Autodesk Inventor part; units mm, degrees
ref_plane "YZ Plane" through (0, 0, 0) normal (1, 0, 0) x (0, 1, 0)
ref_plane "XZ Plane" through (0, 0, 0) normal (0, 1, 0) x (-1, 0, 0)
ref_plane "XY Plane" through (0, 0, 0) normal (0, 0, 1) x (1, 0, 0)
sketch "Sketch1" plane through (0, 0, 0) normal (0, 1, 0) x (-1, 0, 0)
  arc A0 (7, -28.6575) -> (-7, -28.6575) centre (0, 0) ccw
  arc A1 (12.4228, -32.1858) -> (-12.4228, -32.1858) centre (0, 0) ccw
  line L0 (16.5147, 30.2905) -> (25, 38.7758)
  line L1 (16.5147, 30.2905) -> (28.5147, 30.2905) construction
  line L2 (25, 38.7758) -> (-25, 38.7758)
  line L3 (-25, 38.7758) -> (-16.5147, 30.2905)
  line L4 (12.4228, -32.1858) -> (12.4228, -47.1858)
  line L5 (12.4228, -47.1858) -> (7, -47.1858)
  line L6 (7, -47.1858) -> (7, -28.6575)
  line L7 (0, 0) -> (0, -37.5587) construction
  line L8 (-12.4228, -32.1858) -> (-12.4228, -47.1858)
  line L9 (-12.4228, -47.1858) -> (-7, -47.1858)
  line L10 (-7, -47.1858) -> (-7, -28.6575)
  dimension "d0" = 59
  dimension "d5" = 12
  dimension "d6" = 45
  dimension "d7" = 5
  dimension "d15" = 15
  dimension "d46" = 50
  dimension "d47" = 45
  dimension "d48" = 5.4228
  dimension "d49" = 14
  dimension "d50" = 12
extrude "Extrusion3" add sketch "Sketch1" along normal blind 20
sketch "Sketch3" plane through (-25, 0, 38.7758) normal (0, 0, 1) x (1, 0, 0)
  line L0 (0, 0) -> (50, 0)
  line L1 (0, 20) -> (50, 20)
  line L2 (-20, 0) -> (70, 0)
  line L3 (70, 0) -> (70, 20)
  line L4 (70, 20) -> (-20, 20)
  line L5 (-20, 20) -> (-20, 0)
  point P0 (25, 0)
  point P1 (25, 20)
  dimension "d18" = 90
  dimension "d19" = 20
extrude "Extrusion4" add sketch "Sketch3" along normal blind 5
hole "Hole3" at (-12.4228, 10, -39.6858) direction (1, 0, 0) diameter 6 end through all
hole "Hole4" at (-35, 10, 38.7758) direction (0, 0, 1) diameter 6 end through all
hole "Hole5" at (35, 10, 38.7758) direction (0, 0, 1) diameter 6 end through all
properties part number "pumpholder"
Verification items for the finished model (mm, model axes). A direction names the side the tool comes from. Give positions to 0.01 mm unless a question says otherwise; leave off trailing zeros. Order: outer loops, then holes, each group sorted by start corner. A loop starts at its lowest first (then second) coordinate and runs counter-clockwise, first axis right, second up. Notation, with made-up numbers: M 35.5,76.25 L 63.5,76.25 A22 cw 63.5,101.25 Z; hole C 62.25,-11 d8. An arc over 180 degrees is marked long. Answer as a JSON object with one key per item and string values. Group by question number.
1) Cross-section at C-C (x = 0). Enter the section's corners in (y, z).
2) Cross-section at B-B (y = 10). Give the number of separate pieces and of enclosed holes in the cut face, then the cut area to 3 significant figures.
3) Cross-section at D-D (y = 16.75). Enter the section's corners in (x, z).
4) Depth check by flat-ended pin: pin 1 Ø6 at (x, y) = (19.5, 9.5) entering from -Z; pin 2 Ø4 at (y, z) = (15, -16) entering from +X; pin 3 Ø5.5 at (y, z) = (13.5, -33.5) entering from +X. Enter the tip coordinate at first touch or a pass-through.
5) Cross-section at A-A (z = 7.5). Enter the section's corners in (x, y).
6) Mould release check, pull along Y, two halves, no side actions. Record for faces 1 (the face through (0, 20, 32)), 2 (the face through (9.749, 9.099, -36.824)), 3 (the face through (10, 10, -47.186)): released by +Y, released by -Y, zero draft, split by the parting line, or undercut.
7) Scan lines: line 1 along Z through (x, y) = (-9.6, 10); line 2 along X through (y, z) = (4.25, -35); line 3 along Y through (x, z) = (-35, 41.6). Record each from-to range of solid material in increasing order. Write a range as [from, to].
8) Access from +Z, -Z, +X, -X, +Y, -Y to the whole of each face (thin tool, end or side, straight path). Record for faces 4 (the face through (-12.423, 10, -43)), 5 (the face through (32, 10, 41)), 6 (the face through (-20.698, 9.86, 34.474)), 7 (the face through (7, 10, -36)), 8 (the face through (12.423, 10, -43)).
Result sheet:
{
 "1": {"outline": "M 0,29.5 L 20,29.5 L 20,43.78 L 0,43.78 Z"},
 "2": {"separate pieces": "5", "enclosed holes": "0", "area": "1,670 mm2"},
 "3": {"outline": "M -45,38.78 L -25,38.78 L -16.51,30.29 A34.5 ccw -12.42,-32.19 L -12.42,-47.19 L -7,-47.19 L -7,-28.66 A29.5 cw long 7,-28.66 L 7,-47.19 L 12.42,-47.19 L 12.42,-32.19 A34.5 ccw 16.51,30.29 L 25,38.78 L 45,38.78 L 45,43.78 L -45,43.78 Z"},
 "4": {"pin 1": "stops at z = -30.3", "pin 2": "stops at x = 31.53", "pin 3": "stops at x = 15.64"},
 "5": {"outline": "M -33.67,0 L -28.53,0 L -28.53,20 L -33.67,20 Z; M 28.53,0 L 33.67,0 L 33.67,20 L 28.53,20 Z"},
 "6": {"face 1": "released by +Y", "face 2": "undercut", "face 3": "zero draft"},
 "7": {"line 1": "z = [-47.19, -42.69], [-36.69, -27.89], [27.89, 43.78]", "line 2": "x = [-12.42, -7], [7, 12.42]", "line 3": "y = [0, 7], [13, 20]"},
 "8": {"face 4": "-Z, -X, +Y, -Y", "face 5": "+Z", "face 6": "-X, +Y, -Y", "face 7": "-Z, +Y, -Y", "face 8": "-Z, +X, +Y, -Y"}
}
